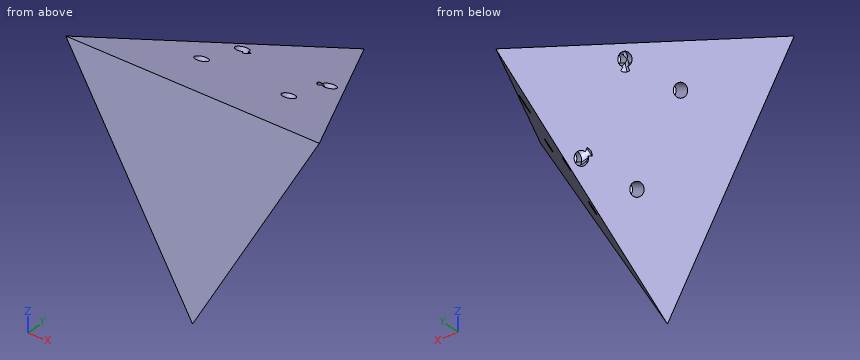
```python
from build123d import *

# Parameters (mm, degrees)
M14X1_5_1_AT_2_COUNT     = 2
M14X1_5_1_AT_2_PITCH     = 86
M14X1_5_1_AT_3_COUNT     = 2
M14X1_5_1_AT_3_PITCH     = 101.548018198
M14X1_5_1_AT_4_COUNT     = 2
M14X1_5_1_AT_4_PITCH     = 54
PATTERN_CIRCULAR_1_COUNT = 3


with BuildPart() as part:
    # 草圖1 → 疊層拉伸1 section 0
    with BuildSketch(Plane(origin=(0, 0, 0), x_dir=(1, 0, 0), z_dir=(0, 1, 0)), mode=Mode.PRIVATE) as loft_1_s0:
        with BuildLine():
            Line((0, 0), (-125, 0))
            Line((-125, 0), (0, 216.506350946))
            Line((0, 216.506350946), (125, 0))
            Line((125, 0), (0, 0))
        make_face()
    loft([loft_1_s0.sketch, Vertex(0, 216.5, -72.168783649)])

    # 草圖3 → M14x1.5 螺紋孔1 (revolve, cut)
    with BuildSketch(Plane(origin=(-43, 117.636383872, -39.21327823), x_dir=(0, -0.9486805150951512, 0.3162361147604725), z_dir=(1, 0, 0))):
        Polygon((0, 0), (0, 23.755378869), (6.25, 20), (6.25, 0), align=None)
    m14x1_5_1 = revolve(axis=Axis((-43, 119.644483201, -33.189156959), (0, -0.31623611476047253, -0.9486805150951512)), mode=Mode.SUBTRACT)

    # M14x1.5 螺紋孔1 at 2: M14x1.5 螺紋孔1 ×2
    with Locations(*[(i * M14X1_5_1_AT_2_PITCH, 0, 0) for i in range(1, M14X1_5_1_AT_2_COUNT)]):
        add(m14x1_5_1, mode=Mode.SUBTRACT)

    # M14x1.5 螺紋孔1 at 3: M14x1.5 螺紋孔1 ×2
    with Locations(*[Vector(0.8468899888530682, -0.5044780658851046, 0.1681642881865052) * (i * M14X1_5_1_AT_3_PITCH) for i in range(1, M14X1_5_1_AT_3_COUNT)]):
        add(m14x1_5_1, mode=Mode.SUBTRACT)

    # M14x1.5 螺紋孔1 at 4: M14x1.5 螺紋孔1 ×2
    with Locations(*[Vector(0, -0.9486805150951512, 0.3162361147604726) * (i * M14X1_5_1_AT_4_PITCH) for i in range(1, M14X1_5_1_AT_4_COUNT)]):
        add(m14x1_5_1, mode=Mode.SUBTRACT)

    # 環狀複製排列1: M14x1.5 螺紋孔1 ×3 about axis
    pattern_circular_1_axis = Axis((0, 216.5, -72.168783649), (0, -1, 0))
    for i in range(1, PATTERN_CIRCULAR_1_COUNT):
        add(m14x1_5_1.rotate(pattern_circular_1_axis, i * 360 / PATTERN_CIRCULAR_1_COUNT), mode=Mode.SUBTRACT)

    # 環狀複製排列1 copy 1 sketch → 環狀複製排列1 copy 1 (revolve, cut)
    with BuildSketch(Plane(origin=(-50.040304887, 117.636383872, -51.407443995), x_dir=(-0.27386850897666026, -0.9486805150951512, -0.15811805738023615), z_dir=(-0.4999999999999998, 0, 0.8660254037844387))):
        Polygon((0, 0), (0, 23.755378869), (6.25, 20), (6.25, 0), align=None)
    revolve(axis=Axis((-55.257346943, 119.644483201, -54.419504631), (0.8215814261477076, -0.31623611476047253, 0.47434025754757536)), mode=Mode.SUBTRACT)

    # 環狀複製排列1 copy 2 sketch → 環狀複製排列1 copy 2 (revolve, cut)
    with BuildSketch(Plane(origin=(7.040304887, 117.636383872, -125.885628721), x_dir=(0.27386850897666015, -0.9486805150951512, -0.15811805738023638), z_dir=(-0.5000000000000004, 0, -0.8660254037844384))):
        Polygon((0, 0), (0, 23.755378869), (6.25, 20), (6.25, 0), align=None)
    revolve(axis=Axis((12.257346943, 119.644483201, -128.897689356), (-0.8215814261477072, -0.31623611476047253, 0.474340257547576)), mode=Mode.SUBTRACT)

    # 環狀複製排列1 copy 3 sketch → 環狀複製排列1 copy 3 (revolve, cut)
    with BuildSketch(Plane(origin=(-64.829204372, 66.407636057, -59.945819094), x_dir=(-0.27386850897666026, -0.9486805150951512, -0.15811805738023615), z_dir=(-0.4999999999999998, 0, 0.8660254037844387))):
        Polygon((0, 0), (0, 23.755378869), (6.25, 20), (6.25, 0), align=None)
    revolve(axis=Axis((-70.046246428, 68.415735385, -62.957879729), (0.8215814261477076, -0.31623611476047253, 0.47434025754757536)), mode=Mode.SUBTRACT)

    # 環狀複製排列1 copy 4 sketch → 環狀複製排列1 copy 4 (revolve, cut)
    with BuildSketch(Plane(origin=(21.829204372, 66.407636057, -134.424003819), x_dir=(0.27386850897666015, -0.9486805150951512, -0.15811805738023638), z_dir=(-0.5000000000000004, 0, -0.8660254037844384))):
        Polygon((0, 0), (0, 23.755378869), (6.25, 20), (6.25, 0), align=None)
    revolve(axis=Axis((27.046246428, 68.415735385, -137.436064455), (-0.8215814261477072, -0.31623611476047253, 0.474340257547576)), mode=Mode.SUBTRACT)

    # 環狀複製排列1 copy 5 sketch → 環狀複製排列1 copy 5 (revolve, cut)
    with BuildSketch(Plane(origin=(-21.829204372, 66.407636057, -134.424003819), x_dir=(-0.27386850897666026, -0.9486805150951512, -0.15811805738023615), z_dir=(-0.4999999999999998, 0, 0.8660254037844387))):
        Polygon((0, 0), (0, 23.755378869), (6.25, 20), (6.25, 0), align=None)
    revolve(axis=Axis((-27.046246428, 68.415735385, -137.436064455), (0.8215814261477076, -0.31623611476047253, 0.47434025754757536)), mode=Mode.SUBTRACT)

    # 環狀複製排列1 copy 6 sketch → 環狀複製排列1 copy 6 (revolve, cut)
    with BuildSketch(Plane(origin=(64.829204372, 66.407636057, -59.945819094), x_dir=(0.27386850897666015, -0.9486805150951512, -0.15811805738023638), z_dir=(-0.5000000000000004, 0, -0.8660254037844384))):
        Polygon((0, 0), (0, 23.755378869), (6.25, 20), (6.25, 0), align=None)
    revolve(axis=Axis((70.046246428, 68.415735385, -62.957879729), (-0.8215814261477072, -0.31623611476047253, 0.474340257547576)), mode=Mode.SUBTRACT)


solid = part.part
```
Source: CAD feature listing. Evaluate the final solid. Frame: model axes, mm. Round coordinates to 2 decimals unless told otherwise and drop trailing zeros. Order: outer loops, then holes, each group sorted by start corner. A loop starts at its lowest first (then second) coordinate and runs counter-clockwise, first axis right, second up. Notation, with made-up numbers: (28, -13) -> (69, -13) arc R25 ccw to (69, 20) -> close; hole circle Ø1 at (47.5, 32). An arc over 180 degrees is marked (long way). Use CSV: the item, a comma, the result in double quotes.
(1) Ray query, L1, parallel to X at y = 128.5, z = -56; L2, parallel to X at y = 160, z = -56; L3, parallel to Z at x = -62.5, y = 94. Return the intervals inside material, ascending.
Report:
L1,"-43.21 to 43.21"
L2,"-31.08 to 31.08"
L3,"-45.58 to -31.33"
(2) Section A-A on x = -88. Return the cut outline in (y, z), and give its area (3 significant figures).
Report:
outline,"(0, -64.09) -> (64.08, -21.36) -> (0, 0) -> close"
area,"2,050 mm^2"
(3) First-contact query: pin 1 Ø1 at (x, y) = (-14, 49.5) entering from +Z; pin 2 Ø12 at (x, y) = (-3, 26) entering from +Z; pin 3 Ø1 at (x, y) = (31.5, 116.5) entering from +Z. Flat tips, straight axial feed; report the tip coordinate or a pass-through.
Report:
pin 1,"z = -16.33"
pin 2,"z = -6.67"
pin 3,"z = -38.67"
(4) Section B-B on y = 33. Return the cut outline in (x, z).
Report:
outline,"(-105.95, -11) -> (0, -194.51) -> (105.95, -11) -> close"
